Build history of the part. All positions in model axes, mm. Face numbers are marked on the shaded views. Round coordinates to 2 decimals unless told otherwise and drop trailing zeros. Write each loop counter-clockwise with the first axis right and the second up, starting at its lowest first coordinate (ties: lowest second). Pieces come first, ordered by that corner, then holes. Notation, with made-up numbers: (30.5, 54) -> (36.5, 54) arc R31 cw to (36.5, 85) -> close; hole circle Ø5 at (-7, 22). An arc over 180 degrees is marked (long way). One line per question, with ' | ' between items.
from build123d import *

# Parameters (mm, degrees)
THREAD1_PITCH           = 2.5
THREAD2_PITCH           = 2.5
SKETCH3_W               = 15
SKETCH3_H               = 10
CUT_EXTRUDE1_DEPTH      = 96.495209461
CUT_EXTRUDE2_DEPTH      = 96.495209461
CUT_EXTRUDE2_DEPTH_BACK = 96.495209461
SKETCH4_W               = 125
SKETCH4_H               = 20.019774924


with BuildPart() as part:
    # Sketch2 → Revolve1 (revolve)
    with BuildSketch(Plane(origin=(0, 0, 0), x_dir=(0, 0, -1), z_dir=(1, 0, 0))):
        Polygon((49.5, 36.15), (47.5, 36.15), (47.5, 12.15), (50, 12.15), (50, 6.65), (60, 6.65), (60, 6.15), (62.5, 6.15), (62.5, 20.15), (60, 20.15), (60, 19.65), (49.5, 19.65), align=None)
    revolve(axis=Axis((0, 0, 0), (0, 1, 0)))

    # Thread1: arcs per turn and ends read off the stored shape
    # Thread1: the profile of Thread Profile1 profile screwed along a right-hand helix through 2.4 turns, 10 arcs to a turn; built about Z, then put on its axis
    thread1_z = Axis((0, 0, 0), (0, 0, 1))
    thread1_corners = [(-40.450607014, -29.389086279, -6.000173205), (-41.326636301, -30.025558812, -5.375000003), (-41.326636301, -30.025558812, -5.125000003), (-40.450607014, -29.389086279, -4.4998268)]
    with BuildLine(mode=Mode.PRIVATE) as thread1_profile:
        Line(thread1_corners[0], thread1_corners[1])
        Line(thread1_corners[1], thread1_corners[2])
        Line(thread1_corners[2], thread1_corners[3])
        Line(thread1_corners[3], thread1_corners[0])
    thread1_cap = Face(thread1_profile.wire())
    thread1_turn_angles = [0, 18, 36, 54, 72, 90, 108, 126, 144, 162, 180, 198, 216, 234, 252, 270, 288, 306, 324, 342, 360]
    thread1_turn_weights = [1, 0.9510565162951535, 1, 0.9510565162951535, 1, 0.9510565162951535, 1, 0.9510565162951535, 1, 0.9510565162951535, 1, 0.9510565162951535, 1, 0.9510565162951535, 1, 0.9510565162951535, 1, 0.9510565162951535, 1, 0.9510565162951535, 1]
    thread1_turn_rails = [Edge.make_bspline([Vector(p[0], p[1], 0).rotate(thread1_z, thread1_turn_angles[k]) / thread1_turn_weights[k] + Vector(0, 0, p[2] + THREAD1_PITCH * thread1_turn_angles[k] / 360) for k in range(21)], [0, 0, 0, 1, 1, 2, 2, 3, 3, 4, 4, 5, 5, 6, 6, 7, 7, 8, 8, 9, 9, 10, 10, 10], 2, thread1_turn_weights) for p in thread1_corners]
    thread1_turn_sides = [Face.make_surface_from_curves(thread1_turn_rails[p[0]], thread1_turn_rails[p[1]]) for p in [(0, 1), (1, 2), (2, 3), (3, 0)]]
    thread1_last_angles = [720, 738, 756, 774, 792, 810, 828, 846, 864]
    thread1_last_weights = [1, 0.9510565162951535, 1, 0.9510565162951535, 1, 0.9510565162951535, 1, 0.9510565162951535, 1]
    thread1_last_rails = [Edge.make_bspline([Vector(p[0], p[1], 0).rotate(thread1_z, thread1_last_angles[k]) / thread1_last_weights[k] + Vector(0, 0, p[2] + THREAD1_PITCH * thread1_last_angles[k] / 360) for k in range(9)], [0, 0, 0, 1, 1, 2, 2, 3, 3, 4, 4, 4], 2, thread1_last_weights) for p in thread1_corners]
    thread1_last_sides = [Face.make_surface_from_curves(thread1_last_rails[p[0]], thread1_last_rails[p[1]]) for p in [(0, 1), (1, 2), (2, 3), (3, 0)]]
    thread1 = Plane(origin=(0, 6.65, 0), x_dir=(1, 0, 0), z_dir=(0, -1, 0)) * Solid(Shell([*[p.moved(Location((0, 0, THREAD1_PITCH * i))) for i in range(2) for p in thread1_turn_sides], *thread1_last_sides, thread1_cap, thread1_cap.rotate(thread1_z, 864).moved(Location((0, 0, THREAD1_PITCH * 864 / 360)))]))
    add(thread1, mode=Mode.SUBTRACT)

    # Thread2: arcs per turn and ends read off the stored shape
    # Thread2: the profile of Thread Profile2 profile screwed along a right-hand helix through 1.6 turns, 10 arcs to a turn; built about Z, then put on its axis
    thread2_z = Axis((0, 0, 0), (0, 0, 1))
    thread2_corners = [(49.4997, 0, -0.000173205), (50.58253175, 0, 0.624999997), (50.58253175, 0, 0.874999997), (49.4997, 0, 1.5001732)]
    with BuildLine(mode=Mode.PRIVATE) as thread2_profile:
        Line(thread2_corners[0], thread2_corners[1])
        Line(thread2_corners[1], thread2_corners[2])
        Line(thread2_corners[2], thread2_corners[3])
        Line(thread2_corners[3], thread2_corners[0])
    thread2_cap = Face(thread2_profile.wire())
    thread2_turn_angles = [0, 18, 36, 54, 72, 90, 108, 126, 144, 162, 180, 198, 216, 234, 252, 270, 288, 306, 324, 342, 360]
    thread2_turn_weights = [1, 0.9510565162951535, 1, 0.9510565162951535, 1, 0.9510565162951535, 1, 0.9510565162951535, 1, 0.9510565162951535, 1, 0.9510565162951535, 1, 0.9510565162951535, 1, 0.9510565162951535, 1, 0.9510565162951535, 1, 0.9510565162951535, 1]
    thread2_turn_rails = [Edge.make_bspline([Vector(p[0], p[1], 0).rotate(thread2_z, thread2_turn_angles[k]) / thread2_turn_weights[k] + Vector(0, 0, p[2] + THREAD2_PITCH * thread2_turn_angles[k] / 360) for k in range(21)], [0, 0, 0, 1, 1, 2, 2, 3, 3, 4, 4, 5, 5, 6, 6, 7, 7, 8, 8, 9, 9, 10, 10, 10], 2, thread2_turn_weights) for p in thread2_corners]
    thread2_turn_sides = [Face.make_surface_from_curves(thread2_turn_rails[p[0]], thread2_turn_rails[p[1]]) for p in [(0, 1), (1, 2), (2, 3), (3, 0)]]
    thread2_last_angles = [360, 378, 396, 414, 432, 450, 468, 486, 504, 522, 540, 558, 576]
    thread2_last_weights = [1, 0.9510565162951535, 1, 0.9510565162951535, 1, 0.9510565162951535, 1, 0.9510565162951535, 1, 0.9510565162951535, 1, 0.9510565162951535, 1]
    thread2_last_rails = [Edge.make_bspline([Vector(p[0], p[1], 0).rotate(thread2_z, thread2_last_angles[k]) / thread2_last_weights[k] + Vector(0, 0, p[2] + THREAD2_PITCH * thread2_last_angles[k] / 360) for k in range(13)], [0, 0, 0, 1, 1, 2, 2, 3, 3, 4, 4, 5, 5, 6, 6, 6], 2, thread2_last_weights) for p in thread2_corners]
    thread2_last_sides = [Face.make_surface_from_curves(thread2_last_rails[p[0]], thread2_last_rails[p[1]]) for p in [(0, 1), (1, 2), (2, 3), (3, 0)]]
    thread2 = Plane(origin=(0, 36.15, 0), x_dir=(-1, 0, 0), z_dir=(0, -1, 0)) * Solid(Shell([*thread2_turn_sides, *thread2_last_sides, thread2_cap, thread2_cap.rotate(thread2_z, 576).moved(Location((0, 0, THREAD2_PITCH * 576 / 360)))]))
    add(thread2)

    # Sketch3 → Cut-Extrude1 (cut, through all)
    with BuildSketch(Plane.XY):
        with Locations((0, 25.587500003)):
            Rectangle(SKETCH3_W, SKETCH3_H)
    extrude(amount=-CUT_EXTRUDE1_DEPTH, mode=Mode.SUBTRACT)

    # Sketch4 → Cut-Extrude2 (cut, two sides: drawn at the far end of the back side and taken through both)
    with BuildSketch(Plane(origin=(0, 0, 0), x_dir=(0, 0, -1), z_dir=(1, 0, 0)).offset(-CUT_EXTRUDE2_DEPTH_BACK)):
        with Locations((0, 30.159887462)):
            Rectangle(SKETCH4_W, SKETCH4_H)
    extrude(amount=CUT_EXTRUDE2_DEPTH + CUT_EXTRUDE2_DEPTH_BACK, mode=Mode.SUBTRACT)


solid = part.part
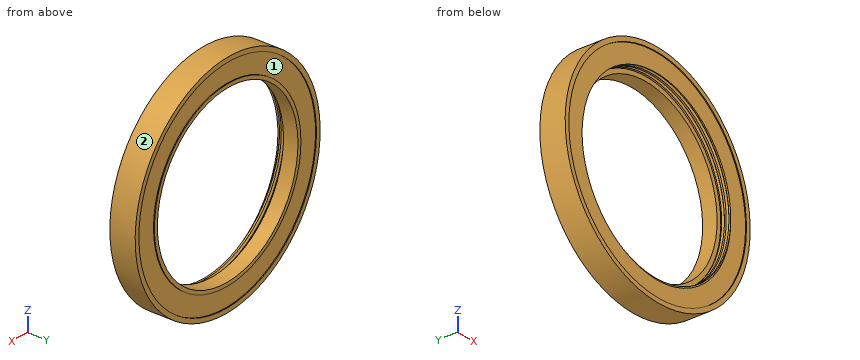
(1) Slice it at B-B (y = 15). Write the cut outline in (x, z), then the cut area to 3 significant figures.
Calculated:
outline: circle Ø125 at (0, 0); hole circle Ø95 at (0, 0) | area: 5,180 mm2
(2) Mould opens along Z. For the marked faces 1 and 2 say: pulls with the +Z half, pulls with the -Z half, needs draft (parallel to the pull), parting line crosses it, or undercut.
Calculated:
face 1: undercut | face 2: parting line crosses it
(3) Wall check: line 1 (X direction, y = 7.1, z = 0); line 2 (X direction, y = 6.55, z = 0); line 3 (Y direction, x = 12, z = 53). Give the ranges that are in metal, low to high. Write a range as from..to.
Calculated:
line 1: -62.5..-51.08, 50..62.5 | line 2: -62.5..-60, 60..62.5 | line 3: 6.65..19.65
(4) Slice it at A-A (x = -53). Write the cut outline in (y, z), then the cut area to 3 significant figures.
Calculated:
outline: (6.15, -33.12) -> (20.15, -33.12) -> (20.15, -28.12) -> (19.65, -28.12) -> (19.65, 28.12) -> (20.15, 28.12) -> (20.15, 33.12) -> (6.15, 33.12) -> (6.15, 28.12) -> (6.65, 28.12) -> (6.65, -28.12) -> (6.15, -28.12) -> close | area: 871 mm2
(5) Drop flat-ended pins along their axis: pin 1 (5 mm diameter, centred on x = 26, y = 17, fed in from +Z); pin 2 (3 mm diameter, centred on x = 45.5, y = 8.5, fed in from +Z); pin 3 (6 mm diameter, centred on x = 27, y = 10.5, fed in from -Z); pin 4 (12 mm diameter, centred on x = 41, z = 0, fed in from +Y). Give the stop position or say it passes through.
Calculated:
pin 1: z = 57.91 | pin 2: z = 44.39 | pin 3: z = -57.71 | pin 4: through
